Build history of the part. All positions in model axes, mm. Give positions to 0.01 mm unless a question says otherwise; leave off trailing zeros. Order: outer loops, then holes, each group sorted by start corner. A loop starts at its lowest first (then second) coordinate and runs counter-clockwise, first axis right, second up. Notation, with made-up numbers: (12.25, 42) -> (37.25, 42) arc R16 ccw to (37.25, 52) -> close; hole circle Ø7 at (18.5, 57). An arc over 180 degrees is marked (long way). Use a Markdown table: item, result. Add a question column.
```python
from build123d import *

# Parameters (mm, degrees)
F0_W     = 127
F0_H     = 190.5
F1_DEPTH = 2.54
F2_W     = 21.605315
F2_H     = 95.25
F3_DEPTH = 2.54
F4_R     = 12.7
F5_DEPTH = 101.870598
F6_R     = 12.7
F6_R_2   = 11.43
F7_DEPTH = 2.54


with BuildPart() as f1:
    # F0 (on Top) → F1 (new body)
    with BuildSketch(Plane.XY):
        Rectangle(F0_W, F0_H)
    extrude(amount=F1_DEPTH)

    # F2 (on face) → F3 (join)
    with BuildSketch(Plane.XY.offset(2.54)):
        with Locations((74.302657, -47.625)):
            Rectangle(F2_W, F2_H)
    extrude(amount=-F3_DEPTH)

    # F4 (on face) → F5 (cut)
    with BuildSketch(Plane.XY.offset(2.54)):
        with Locations((40.655315, -50.8)):
            Circle(F4_R)
    extrude(amount=-F5_DEPTH, mode=Mode.SUBTRACT)

    # F6 (on face) → F7 (join)
    with BuildSketch(Plane.XY.offset(2.54)):
        with Locations((40.655315, -50.8)):
            Circle(F6_R)
        with Locations((40.655315, -50.8)):
            Circle(F6_R_2, mode=Mode.SUBTRACT)
    extrude(amount=-F7_DEPTH)


solid = f1.part
```
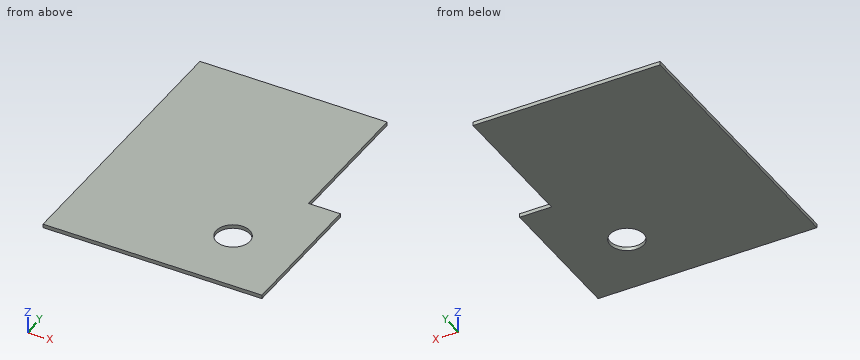
(1) Band-saw the part on A-A on y = -50.8. Give the cut face in (x, z).
(2) Band-saw the part on B-B on x = 33. Give the cut face in (y, z).
(3) Band-saw the part on C-C on z = 1.65. Give the cut face in (x, y), plus the area to 3 significant figures.
(4) Band-saw the part on D-D on y = 39. Give the cut face in (x, z), plus the area to 3 significant figures.
(5) Wall check: probe 1 along X at (y, z) = (48, 0.85); probe 2 along Y at (x, z) = (31, 1.9); probe 3 along Y at (x, z) = (45, 1.5). Give the ranges that are in metal, low to high.
(6) Pin check, flat tip, straight feed: pin 1 Ø1.3 at (x, z) = (75, 0.5) entering from +Y. Stop position of the tip, or through.
Response:
| question | item | result |
|---|---|---|
| 1 | outline | (-63.5, 0) -> (29.23, 0) -> (29.23, 2.54) -> (-63.5, 2.54) -> close; (52.09, 0) -> (85.11, 0) -> (85.11, 2.54) -> (52.09, 2.54) -> close |
| 2 | outline | (-95.25, 0) -> (-59.29, 0) -> (-59.29, 2.54) -> (-95.25, 2.54) -> close; (-42.31, 0) -> (95.25, 0) -> (95.25, 2.54) -> (-42.31, 2.54) -> close |
| 3 | outline | (-63.5, -95.25) -> (85.11, -95.25) -> (85.11, 0) -> (63.5, 0) -> (63.5, 95.25) -> (-63.5, 95.25) -> close; hole circle Ø22.86 at (40.66, -50.8) |
| 3 | area | 25,800 mm² |
| 4 | outline | (-63.5, 0) -> (63.5, 0) -> (63.5, 2.54) -> (-63.5, 2.54) -> close |
| 4 | area | 323 mm² |
| 5 | probe 1 | x = -63.5 to 63.5 |
| 5 | probe 2 | y = -95.25 to -56.92, -44.68 to 95.25 |
| 5 | probe 3 | y = -95.25 to -61.37, -40.23 to 95.25 |
| 6 | pin 1 | stops at y = 0 |
